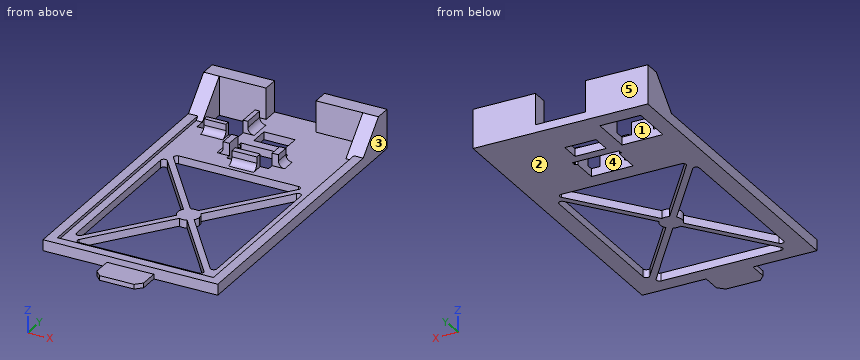
```python
from build123d import *

# Parameters (mm, degrees)
SKETCH1_W            = 56
SKETCH1_H            = 100
BOSS_EXTRUDE1_DEPTH  = 2.5
SKETCH2_W            = 20
SKETCH2_H            = 5.05
BOSS_EXTRUDE2_DEPTH  = 10
SKETCH3_W            = 13.1
SKETCH3_H            = 13.1
CUT_EXTRUDE1_DEPTH   = 112.005866962
BOSS_EXTRUDE3_DEPTH  = 5
BOSS_EXTRUDE4_DEPTH  = 5
SKETCH6_W            = 7
SKETCH6_H            = 1.5
SKETCH6_W_2          = 1.5
SKETCH6_H_2          = 7
BOSS_EXTRUDE5_DEPTH  = 4
SKETCH7_W            = 15
SKETCH7_H            = 1.3
CUT_EXTRUDE2_DEPTH   = 112.005866962
SKETCH8_W            = 13.4
SKETCH8_H            = 8.5
SKETCH8_W_2          = 10
SKETCH8_H_2          = 6
CUT_EXTRUDE3_DEPTH   = 112.005866962
FILLET1_R            = 2
SKETCH9_W            = 15
SKETCH9_H            = 8
BOSS_EXTRUDE6_DEPTH  = 2.5
CHAMFER1_SIZE        = 2
SKETCH10_W           = 45
SKETCH10_H           = 59
CUT_EXTRUDE4_DEPTH   = 4
BOSS_EXTRUDE7_DEPTH  = 2.5
FILLET2_R            = 1
FILLET3_R            = 0.5
CUT_EXTRUDE5_DEPTH   = 1
SKETCH13_W           = 1
SKETCH13_H           = 88
BOSS_EXTRUDE8_DEPTH  = 3
BOSS_EXTRUDE9_DEPTH  = 3
SKETCH15_W           = 50
SKETCH15_H           = 3
BOSS_EXTRUDE10_DEPTH = 1
SKETCH16_W           = 2
SKETCH16_H           = 5
SKETCH16_W_2         = 8
SKETCH16_H_2         = 2
SKETCH16_H_3         = 4.4346707
BOSS_EXTRUDE11_DEPTH = 4
FILLET4_R            = 2


with BuildPart() as part:
    # Sketch1 → Boss-Extrude1 (new body)
    with BuildSketch(Plane.XY):
        with Locations((0, -56.95)):
            Rectangle(SKETCH1_W, SKETCH1_H)
    extrude(amount=BOSS_EXTRUDE1_DEPTH)

    # Sketch2 → Boss-Extrude2 (add)
    with BuildSketch(Plane.XY.offset(2.5)):
        with Locations((-18, -9.475)):
            Rectangle(SKETCH2_W, SKETCH2_H)
        with Locations((18, -9.475)):
            Rectangle(SKETCH2_W, SKETCH2_H)
    extrude(amount=BOSS_EXTRUDE2_DEPTH)

    # Sketch3 → Cut-Extrude1 (cut, through all)
    with BuildSketch(Plane.XY.offset(2.5)):
        with Locations((-16.45, -18.55)):
            Rectangle(SKETCH3_W, SKETCH3_H)
    extrude(amount=-CUT_EXTRUDE1_DEPTH, mode=Mode.SUBTRACT)

    # Sketch4 → Boss-Extrude3 (add)
    with BuildSketch(Plane(origin=(28, 0, 0), x_dir=(0, 0, -1), z_dir=(1, 0, 0))):
        Polygon((-12.5, -12), (-2.5, -12), (-2.5, -22), align=None)
    extrude(amount=-BOSS_EXTRUDE3_DEPTH)

    # Sketch5 → Boss-Extrude4 (add)
    with BuildSketch(Plane.ZY.offset(28)):
        Polygon((2.5, -22), (12.5, -12), (2.5, -12), align=None)
    extrude(amount=-BOSS_EXTRUDE4_DEPTH)

    # Sketch6 → Boss-Extrude5 (add)
    with BuildSketch(Plane.XY.offset(2.5)):
        with Locations((-16.45, -25.85)):
            Rectangle(SKETCH6_W, SKETCH6_H)
        with Locations((-9.15, -18.55)):
            Rectangle(SKETCH6_W_2, SKETCH6_H_2)
    extrude(amount=BOSS_EXTRUDE5_DEPTH)

    # Sketch7 → Cut-Extrude2 (cut, through all)
    with BuildSketch(Plane.XY.offset(2.5)):
        with Locations((0, -28.45)):
            Rectangle(SKETCH7_W, SKETCH7_H)
    extrude(amount=-CUT_EXTRUDE2_DEPTH, mode=Mode.SUBTRACT)

    # Sketch8 → Cut-Extrude3 (cut, through all)
    with BuildSketch(Plane.XY.offset(2.5)):
        with Locations((0, -33.35)):
            Rectangle(SKETCH8_W, SKETCH8_H)
        with Locations((0, -21.8)):
            Rectangle(SKETCH8_W_2, SKETCH8_H_2)
    extrude(amount=-CUT_EXTRUDE3_DEPTH, mode=Mode.SUBTRACT)

    # Fillet1
    fillet1_edges = [part.edges().sort_by_distance(p)[0] for p in [
        (-16.45, -26.6, 2.5),
        (-8.4, -18.55, 2.5),
    ]]
    fillet(fillet1_edges, radius=FILLET1_R)

    # Sketch9 → Boss-Extrude6 (add)
    with BuildSketch(Plane.XY.offset(2.5)):
        with Locations((0, -110.95)):
            Rectangle(SKETCH9_W, SKETCH9_H)
    extrude(amount=-BOSS_EXTRUDE6_DEPTH)

    # Chamfer1
    chamfer1_edges = [part.edges().sort_by_distance(p)[0] for p in [
        (-7.5, -114.95, 1.25),
        (7.5, -114.95, 1.25),
    ]]
    chamfer(chamfer1_edges, length=CHAMFER1_SIZE)

    # Sketch10 → Cut-Extrude4 (cut)
    with BuildSketch(Plane.XY.offset(2.5)):
        with Locations((0, -72.45)):
            Rectangle(SKETCH10_W, SKETCH10_H)
    extrude(amount=-CUT_EXTRUDE4_DEPTH, mode=Mode.SUBTRACT)

    # Sketch11 → Boss-Extrude7 (add)
    with BuildSketch(Plane.XY.offset(2.5)):
        with BuildLine():
            Line((-21.242331765, -42.95), (-22.5, -42.95))
            Line((-22.5, -42.95), (-22.5, -44.598942796))
            Line((-22.5, -44.598942796), (-2.829214626, -70.389528064))
            ThreePointArc((-2.829214626, -70.389528064), (-2.122572116, -69.667072115), (-1.238970121, -69.176629712))
            Line((-1.238970121, -69.176629712), (-21.242331765, -42.95))
        make_face()
        with BuildLine():
            Line((22.5, -42.95), (21.242331765, -42.95))
            Line((21.242331765, -42.95), (1.238970121, -69.176629712))
            ThreePointArc((1.238970121, -69.176629712), (2.122572116, -69.667072115), (2.829214626, -70.389528064))
            Line((2.829214626, -70.389528064), (22.5, -44.598942796))
            Line((22.5, -44.598942796), (22.5, -42.95))
        make_face()
        with BuildLine():
            Line((22.5, -100.301057204), (2.829214626, -74.510471936))
            ThreePointArc((2.829214626, -74.510471936), (2.122572116, -75.232927885), (1.238970121, -75.723370288))
            Line((1.238970121, -75.723370288), (21.242331765, -101.95))
            Line((21.242331765, -101.95), (22.5, -101.95))
            Line((22.5, -101.95), (22.5, -100.301057204))
        make_face()
        with BuildLine():
            Line((-2.829214626, -74.510471936), (-22.5, -100.301057204))
            Line((-22.5, -100.301057204), (-22.5, -101.95))
            Line((-22.5, -101.95), (-21.242331765, -101.95))
            Line((-21.242331765, -101.95), (-1.238970121, -75.723370288))
            ThreePointArc((-1.238970121, -75.723370288), (-2.122572116, -75.232927885), (-2.829214626, -74.510471936))
        make_face()
        with BuildLine():
            Line((-1.257668235, -72.45), (-2.829214626, -70.389528064))
            ThreePointArc((-2.829214626, -70.389528064), (-3.5, -72.45), (-2.829214626, -74.510471936))
            Line((-2.829214626, -74.510471936), (-1.257668235, -72.45))
        make_face()
        with BuildLine():
            Line((0, -70.801057204), (-1.238970121, -69.176629712))
            ThreePointArc((-1.238970121, -69.176629712), (-2.122572116, -69.667072115), (-2.829214626, -70.389528064))
            Line((-2.829214626, -70.389528064), (-1.257668235, -72.45))
            Line((-1.257668235, -72.45), (0, -70.801057204))
        make_face()
        with BuildLine():
            Line((0, -74.098942796), (-1.257668235, -72.45))
            Line((-1.257668235, -72.45), (-2.829214626, -74.510471936))
            ThreePointArc((-2.829214626, -74.510471936), (-2.122572116, -75.232927885), (-1.238970121, -75.723370288))
            Line((-1.238970121, -75.723370288), (0, -74.098942796))
        make_face()
        with BuildLine():
            Line((1.238970121, -75.723370288), (0, -74.098942796))
            Line((0, -74.098942796), (-1.238970121, -75.723370288))
            ThreePointArc((-1.238970121, -75.723370288), (0, -75.95), (1.238970121, -75.723370288))
        make_face()
        with BuildLine():
            Line((2.829214626, -70.389528064), (1.257668235, -72.45))
            Line((1.257668235, -72.45), (2.829214626, -74.510471936))
            ThreePointArc((2.829214626, -74.510471936), (3.328081369, -73.533454846), (3.5, -72.45))
            ThreePointArc((3.5, -72.45), (3.328081369, -71.366545154), (2.829214626, -70.389528064))
        make_face()
        with BuildLine():
            Line((2.829214626, -74.510471936), (1.257668235, -72.45))
            Line((1.257668235, -72.45), (0, -74.098942796))
            Line((0, -74.098942796), (1.238970121, -75.723370288))
            ThreePointArc((1.238970121, -75.723370288), (2.122572116, -75.232927885), (2.829214626, -74.510471936))
        make_face()
        with BuildLine():
            Line((1.238970121, -69.176629712), (0, -70.801057204))
            Line((0, -70.801057204), (1.257668235, -72.45))
            Line((1.257668235, -72.45), (2.829214626, -70.389528064))
            ThreePointArc((2.829214626, -70.389528064), (2.122572116, -69.667072115), (1.238970121, -69.176629712))
        make_face()
        with BuildLine():
            ThreePointArc((1.238970121, -69.176629712), (0, -68.95), (-1.238970121, -69.176629712))
            Line((-1.238970121, -69.176629712), (0, -70.801057204))
            Line((0, -70.801057204), (1.238970121, -69.176629712))
        make_face()
        Polygon((1.257668235, -72.45), (0, -70.801057204), (-1.257668235, -72.45), (0, -74.098942796), align=None)
    extrude(amount=-BOSS_EXTRUDE7_DEPTH)

    # Fillet2
    fillet2_edges = [part.edges().sort_by_distance(p)[0] for p in [
        (-22.5, -100.301057204, 1.25),
        (-21.242331765, -101.95, 1.25),
        (21.242331765, -101.95, 1.25),
        (22.5, -100.301057204, 1.25),
        (22.5, -44.598942796, 1.25),
        (21.242331765, -42.95, 1.25),
        (-21.242331765, -42.95, 1.25),
        (-22.5, -44.598942796, 1.25),
    ]]
    fillet(fillet2_edges, radius=FILLET2_R)

    # Fillet3
    fillet3_edges = [part.edges().sort_by_distance(p)[0] for p in [
        (6.7, -29.1, 1.25),
        (-6.7, -29.1, 1.25),
    ]]
    fillet(fillet3_edges, radius=FILLET3_R)

    # Sketch12 → Cut-Extrude5 (cut)
    with BuildSketch(Plane.XY.offset(2.5)):
        Polygon((-7.5, -106.95), (7.5, -106.95), (7.5, -112.95), (5.5, -114.95), (-5.5, -114.95), (-7.5, -112.95), align=None)
    extrude(amount=-CUT_EXTRUDE5_DEPTH, mode=Mode.SUBTRACT)

    # Sketch13 → Boss-Extrude8 (add)
    with BuildSketch(Plane(origin=(28, 0, 0), x_dir=(0, 0, -1), z_dir=(1, 0, 0))):
        with Locations((-3, -62.95)):
            Rectangle(SKETCH13_W, SKETCH13_H)
    extrude(amount=-BOSS_EXTRUDE8_DEPTH)

    # Sketch14 → Boss-Extrude9 (add)
    with BuildSketch(Plane.ZY.offset(28)):
        Polygon((3.5, -21), (3.5, -106.95), (2.5, -106.95), (2.5, -22), align=None)
    extrude(amount=-BOSS_EXTRUDE9_DEPTH)

    # Sketch15 → Boss-Extrude10 (add)
    with BuildSketch(Plane.XY.offset(2.5)):
        with Locations((0, -105.45)):
            Rectangle(SKETCH15_W, SKETCH15_H)
    extrude(amount=BOSS_EXTRUDE10_DEPTH)

    # Sketch16 → Boss-Extrude11 (add)
    with BuildSketch(Plane.XY.offset(2.5)):
        with Locations((-7.7, -33.6)):
            Rectangle(SKETCH16_W, SKETCH16_H)
        with Locations((0, -38.6)):
            Rectangle(SKETCH16_W_2, SKETCH16_H_2)
        with Locations((7.7, -33.31733535)):
            Rectangle(SKETCH16_W, SKETCH16_H_3)
    extrude(amount=BOSS_EXTRUDE11_DEPTH)

    # Fillet4
    fillet4_edges = [part.edges().sort_by_distance(p)[0] for p in [
        (-8.7, -33.6, 2.5),
        (0, -39.6, 2.5),
        (8.7, -33.31733535, 2.5),
    ]]
    fillet(fillet4_edges, radius=FILLET4_R)


solid = part.part
```
The listing builds one solid part. Answer for the finished solid, in the listing's coordinates (mm). Face numbers are marked on the shaded views. A direction names the side the tool comes from. Coordinates: 2 decimals unless noted, no trailing zeros. Loops run counter-clockwise (first coordinate to the right, second up) from the corner with the lowest first, then second, coordinate; pieces in that order, holes last. Notation, with made-up numbers: M 28.5,27.25 L 69.5,27.25 A31 ccw 69.5,52.25 Z; hole C -27.75,59 d1. An arc over 180 degrees is marked long. Answer as a JSON object with one key per item and string values. Group by question number.
Item 1: Determine the mould class of the marked faces 3, 4 and 5 for opening direction X: +X half, -X half, draft (parallel to the pull), parting line (faces both ways), or undercut.
Item 2: Section B-B (x = 14.5) is taken. Write down the section's boundary in (y, z), and give its area (3 significant figures).
Item 3: Consider L1, parallel to X at y = -93.5, z = 3; L2, parallel to Y at x = 22, z = 3.25; L3, parallel to X at y = -31.5, z = 1. Determine where each line is inside the solid, lowest interval first.
Item 4: Which of the six approach directions +Z, -Z, +X, -X, +Y, -Y give full straight-line access (tool end or side, diameter ignored) to the marked faces 1 and 2?
Item 5: Section A-A (z = 8) is taken. Write down the section's boundary in (x, y).
Item 6: Each of these flat-tipped pins is pushed along its axis until it touches: P1, Ø2, axis at y = -33.5, z = 5.5, coming from the +X side; P2, Ø3, axis at x = 18, y = -92, coming from the -Z side; P3, Ø1, axis at x = -7.5, z = 5, coming from the -Y side; P4, Ø1.2, axis at y = -108.5, z = 1, coming from the +X side. Where does it stop, or does it pass through?
Item 7: Section C-C (y = -93.5) is taken. Write down the section's boundary in (x, z), and give its area (3 significant figures).
Solved:
{
 "1": {"face 3": "+X half", "face 4": "undercut", "face 5": "draft"},
 "2": {"outline": "M -106.95,0 L -101.95,0 L -101.95,2.5 L -103.95,2.5 L -103.95,3.5 L -106.95,3.5 Z; M -93.11,0 L -89.81,0 L -89.81,2.5 L -93.11,2.5 Z; M -55.09,0 L -51.79,0 L -51.79,2.5 L -55.09,2.5 Z; M -42.95,0 L -6.95,0 L -6.95,12.5 L -12,12.5 L -12,2.5 L -42.95,2.5 Z", "area": "172 mm2"},
 "3": {"L1": "x = -28 to -25, 25 to 28", "L2": "y = -106.95 to -103.95, -12 to -6.95", "L3": "x = -28 to -6.7, 6.7 to 28"},
 "4": {"face 1": "+Z, -Z", "face 2": "-Z, +X, -X, +Y, -Y"},
 "5": {"outline": "M -28,-16.5 L -23,-16.5 L -23,-12 L -8,-12 L -8,-6.95 L -28,-6.95 Z; M 8,-12 L 23,-12 L 23,-16.5 L 28,-16.5 L 28,-6.95 L 8,-6.95 Z"},
 "6": {"P1": "stops at x = 8.7", "P2": "stops at z = 0", "P3": "stops at y = -36.1", "P4": "stops at x = 7.5"},
 "7": {"outline": "M -28,0 L -22.5,0 L -22.5,2.5 L -25,2.5 L -25,3.5 L -28,3.5 Z; M -17.31,0 L -14.8,0 L -14.8,2.5 L -17.31,2.5 Z; M 14.8,0 L 17.31,0 L 17.31,2.5 L 14.8,2.5 Z; M 22.5,0 L 28,0 L 28,3.5 L 25,3.5 L 25,2.5 L 22.5,2.5 Z", "area": "46.1 mm2"}
}
